Source: three-view drawing plus pictorial views. Frame: mm from the lowest corner of the part. Coordinates: 2 decimals unless noted, no trailing zeros. Write each loop counter-clockwise with the first axis right and the second up, starting at its lowest first coordinate (ties: lowest second). Pieces come first, ordered by that corner, then holes. Notation, with made-up numbers: (52.5, 28.25) -> (108.5, 28.25) arc R28 cw to (108.5, 67.25) -> close; hole circle Ø9 at (21, 60). An arc over 180 degrees is marked (long way). One line per item, written item: value.
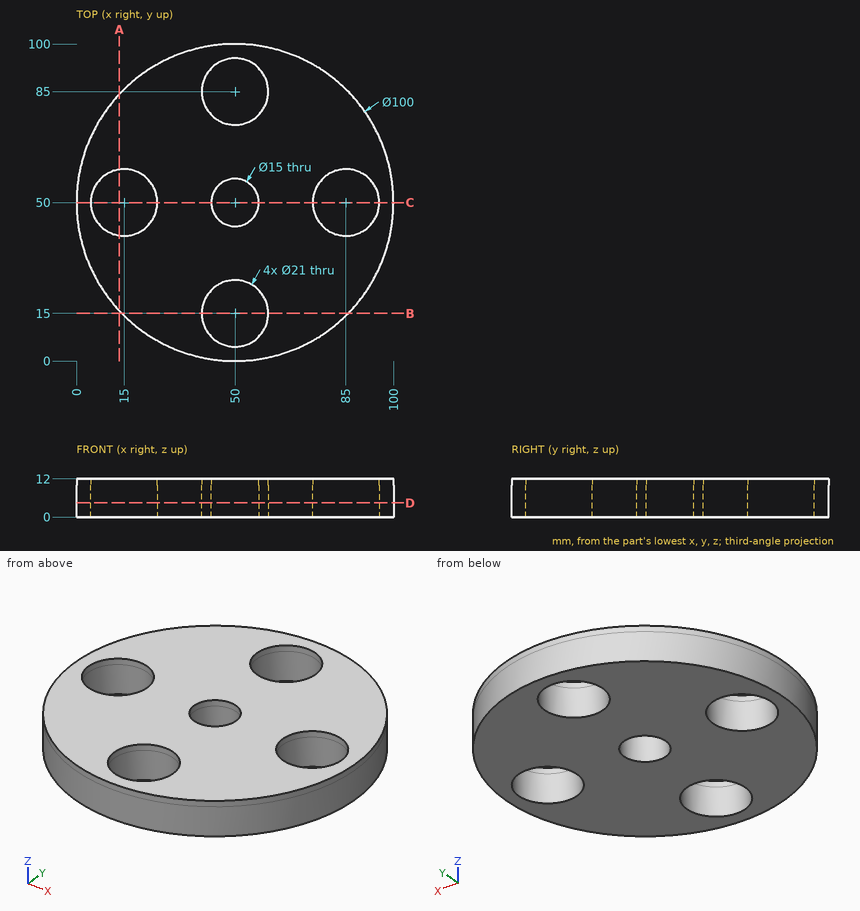
(1) First-contact query: pin 1 (17 mm diameter, centred on x = 50, y = 85, fed in from +Z); pin 2 (4 mm diameter, centred on x = 77.5, z = 4, fed in from +Y); pin 3 (6 mm diameter, centred on x = 23.5, z = 2, fed in from -Y); pin 4 (6 mm diameter, centred on y = 22, z = 10, fed in from -X). Flat tips, straight axial feed; report the tip coordinate or a pass-through.
Responses:
pin 1: passes through
pin 2: stops at y = 93.01
pin 3: stops at y = 5.87
pin 4: stops at x = 6.7
(2) Section C-C (y = 50). Return the cut outline in (x, z).
Responses:
outline: (0, 0) -> (4.5, 0) -> (4.5, 12) -> (0, 12) -> close; (25.5, 0) -> (42.5, 0) -> (42.5, 12) -> (25.5, 12) -> close; (57.5, 0) -> (74.5, 0) -> (74.5, 12) -> (57.5, 12) -> close; (95.5, 0) -> (100, 0) -> (100, 12) -> (95.5, 12) -> close
(3) Line query: line 1 (Y direction, x = 50, z = 11.4); line 2 (X direction, y = 45, z = 8); line 3 (X direction, y = 44, z = 8.75). Output: solid intervals per line, ascending. Write a range as [from, to].
Responses:
line 1: y = [0, 4.5], [25.5, 42.5], [57.5, 74.5], [95.5, 100]
line 2: x = [0.25, 5.77], [24.23, 44.41], [55.59, 75.77], [94.23, 99.75]
line 3: x = [0.36, 6.38], [23.62, 45.5], [54.5, 76.38], [93.62, 99.64]
(4) Section A-A (x = 13.5). Return the cut outline in (y, z), then the cut area to 3 significant figures.
Responses:
outline: (15.83, 0) -> (39.61, 0) -> (39.61, 12) -> (15.83, 12) -> close; (60.39, 0) -> (84.17, 0) -> (84.17, 12) -> (60.39, 12) -> close
area: 571 mm2
(5) Section D-D (z = 4.5). Return the cut outline in (x, y).
Responses:
outline: circle Ø100 at (50, 50); hole circle Ø21 at (15, 50); hole circle Ø21 at (50, 15); hole circle Ø21 at (50, 85); hole circle Ø15 at (50, 50); hole circle Ø21 at (85, 50)
(6) Section B-B (y = 15). Return the cut outline in (x, z).
Responses:
outline: (14.29, 0) -> (39.5, 0) -> (39.5, 12) -> (14.29, 12) -> close; (60.5, 0) -> (85.71, 0) -> (85.71, 12) -> (60.5, 12) -> close
